The listing builds one solid part. Answer for the finished solid, in the listing's coordinates (mm). A direction names the side the tool comes from. Round coordinates to 2 decimals unless told otherwise and drop trailing zeros. Loops run counter-clockwise (first coordinate to the right, second up) from the corner with the lowest first, then second, coordinate; pieces in that order, holes last. Notation, with made-up numbers: M 70.5,58 L 90.5,58 A8 ccw 90.5,68 Z; hole C 86,67 d11. An arc over 180 degrees is marked long. Answer as a JSON object with one key per item and string values.
```python
from build123d import *

# Parameters (mm, degrees)
BOSS_EXTRUDE1_DEPTH     = 13
SKETCH6_W               = 6
SKETCH6_H               = 5
BOSS_EXTRUDE4_DEPTH     = 5.6
SKETCH16_W              = 6
SKETCH16_H              = 8
BOSS_EXTRUDE5_DEPTH     = 0.1
CUT_EXTRUDE6_DEPTH      = 4
CUT_EXTRUDE6_DEPTH_BACK = 3.6
SKETCH15_R              = 1.2
CUT_EXTRUDE7_DEPTH      = 8.7202
CUT_EXTRUDE8_START      = -0.2202
SKETCH19_W              = 6
SKETCH19_H              = 8
SKETCH19_R              = 1.2
CUT_EXTRUDE8_DEPTH      = 0.2202
SKETCH12_R              = 1.2
CUT_EXTRUDE5_DEPTH      = 6
CHAMFER1_SIZE           = 0.2
SKETCH21_R              = 1.2
BOSS_EXTRUDE6_DEPTH     = 2.5
SKETCH24_W              = 6
SKETCH24_H              = 5.5
CUT_EXTRUDE10_DEPTH     = 8.5
SKETCH25_W              = 6
SKETCH25_H              = 7
BOSS_EXTRUDE8_DEPTH     = 12.9
SKETCH26_W              = 6
SKETCH26_H              = 7.39
BOSS_EXTRUDE9_DEPTH     = 5
SKETCH27_W              = 6
SKETCH27_H              = 7.39
BOSS_EXTRUDE10_DEPTH    = 8
SKETCH28_R              = 1.2
CUT_EXTRUDE11_DEPTH     = 7.5
SKETCH30_R              = 1.2
CUT_EXTRUDE13_DEPTH     = 8
SKETCH31_W              = 7
SKETCH31_H              = 12.9
BOSS_EXTRUDE11_DEPTH    = 0.5
SKETCH32_W              = 7
SKETCH32_H              = 12.9
BOSS_EXTRUDE12_DEPTH    = 0.5
SKETCH33_W              = 0.5
SKETCH33_H              = 7.39
BOSS_EXTRUDE13_DEPTH    = 13
SKETCH34_R              = 1.2
CUT_EXTRUDE14_DEPTH     = 5


with BuildPart() as part:
    # Sketch1 → Boss-Extrude1 (new body)
    with BuildSketch(Plane.XY):
        Polygon((3, 3.05), (3, -2.253801214), (2.388188946, -2.95), (-2.388188946, -2.95), (-3, -2.253801214), (-3, 3.05), align=None)
    extrude(amount=BOSS_EXTRUDE1_DEPTH)

    # Sketch6 → Boss-Extrude4 (add)
    with BuildSketch(Plane(origin=(0, 3.05, 0), x_dir=(1, 0, 0), z_dir=(0, 1, 0))):
        with Locations((0, -2.5)):
            Rectangle(SKETCH6_W, SKETCH6_H)
    extrude(amount=BOSS_EXTRUDE4_DEPTH)

    # Sketch16 → Boss-Extrude5 (add)
    with BuildSketch(Plane(origin=(0, 3.05, 0), x_dir=(1, 0, 0), z_dir=(0, 1, 0))):
        with Locations((0, -9)):
            Rectangle(SKETCH16_W, SKETCH16_H)
    extrude(amount=BOSS_EXTRUDE5_DEPTH)

    # Sketch18 → Cut-Extrude6 (cut, two sides: drawn at the far end of the back side and taken through both)
    with BuildSketch(Plane(origin=(0, 0, 0), x_dir=(0, 0, -1), z_dir=(1, 0, 0)).offset(-CUT_EXTRUDE6_DEPTH_BACK)):
        with BuildLine():
            Line((-8.8572, -0.0702), (-12.8572, -0.0702))
            Line((-12.8572, -0.0702), (-13, -0.0702))
            Line((-13, -0.0702), (-13, -0.7))
            Line((-13, -0.7), (-12.8572, -0.7))
            Line((-12.8572, -0.7), (-12.7144, -0.7))
            add(Edge.make_bspline(
                [(-12.7144, -0.7), (-12.5198, -0.7), (-12.43, -0.9509)],
                knots=[0.103448276, 0.103448276, 0.103448276, 0.137931034, 0.137931034, 0.137931034], degree=2))
            add(Edge.make_bspline(
                [(-12.43, -0.9509), (-12.3594, -1.2388), (-12.13, -1.45), (-11.8572, -1.45)],
                knots=[0.137931034, 0.137931034, 0.137931034, 0.137931034, 0.172413793, 0.172413793, 0.172413793, 0.172413793], degree=3))
            add(Edge.make_bspline(
                [(-11.8572, -1.45), (-11.5844, -1.45), (-11.355, -1.2388), (-11.2844, -0.9509)],
                knots=[0.172413793, 0.172413793, 0.172413793, 0.172413793, 0.206896552, 0.206896552, 0.206896552, 0.206896552], degree=3))
            add(Edge.make_bspline(
                [(-11.2844, -0.9509), (-11.1946, -0.7), (-11, -0.7)],
                knots=[0.206896552, 0.206896552, 0.206896552, 0.24137931, 0.24137931, 0.24137931], degree=2))
            Line((-11, -0.7), (-10.8572, -0.7))
            Line((-10.8572, -0.7), (-10.7144, -0.7))
            add(Edge.make_bspline(
                [(-10.7144, -0.7), (-10.5198, -0.7), (-10.43, -0.9509)],
                knots=[0.310344828, 0.310344828, 0.310344828, 0.344827586, 0.344827586, 0.344827586], degree=2))
            add(Edge.make_bspline(
                [(-10.43, -0.9509), (-10.3594, -1.2388), (-10.13, -1.45), (-9.8572, -1.45)],
                knots=[0.344827586, 0.344827586, 0.344827586, 0.344827586, 0.379310345, 0.379310345, 0.379310345, 0.379310345], degree=3))
            add(Edge.make_bspline(
                [(-9.8572, -1.45), (-9.5844, -1.45), (-9.355, -1.2388), (-9.2844, -0.9509)],
                knots=[0.379310345, 0.379310345, 0.379310345, 0.379310345, 0.413793103, 0.413793103, 0.413793103, 0.413793103], degree=3))
            add(Edge.make_bspline(
                [(-9.2844, -0.9509), (-9.1946, -0.7), (-9, -0.7)],
                knots=[0.413793103, 0.413793103, 0.413793103, 0.448275862, 0.448275862, 0.448275862], degree=2))
            Line((-9, -0.7), (-8.8572, -0.7))
            Line((-8.8572, -0.7), (-8.7144, -0.7))
            add(Edge.make_bspline(
                [(-8.7144, -0.7), (-8.5198, -0.7), (-8.43, -0.9509)],
                knots=[0.517241379, 0.517241379, 0.517241379, 0.551724138, 0.551724138, 0.551724138], degree=2))
            add(Edge.make_bspline(
                [(-8.43, -0.9509), (-8.3594, -1.2388), (-8.13, -1.45), (-7.8572, -1.45)],
                knots=[0.551724138, 0.551724138, 0.551724138, 0.551724138, 0.586206897, 0.586206897, 0.586206897, 0.586206897], degree=3))
            add(Edge.make_bspline(
                [(-7.8572, -1.45), (-7.5844, -1.45), (-7.355, -1.2388), (-7.2844, -0.9509)],
                knots=[0.586206897, 0.586206897, 0.586206897, 0.586206897, 0.620689655, 0.620689655, 0.620689655, 0.620689655], degree=3))
            add(Edge.make_bspline(
                [(-7.2844, -0.9509), (-7.1946, -0.7), (-7, -0.7)],
                knots=[0.620689655, 0.620689655, 0.620689655, 0.655172414, 0.655172414, 0.655172414], degree=2))
            Line((-7, -0.7), (-6.8572, -0.7))
            Line((-6.8572, -0.7), (-6.7144, -0.7))
            add(Edge.make_bspline(
                [(-6.7144, -0.7), (-6.5198, -0.7), (-6.43, -0.9509)],
                knots=[0.724137931, 0.724137931, 0.724137931, 0.75862069, 0.75862069, 0.75862069], degree=2))
            add(Edge.make_bspline(
                [(-6.43, -0.9509), (-6.3594, -1.2388), (-6.13, -1.45), (-5.8572, -1.45)],
                knots=[0.75862069, 0.75862069, 0.75862069, 0.75862069, 0.793103448, 0.793103448, 0.793103448, 0.793103448], degree=3))
            add(Edge.make_bspline(
                [(-5.8572, -1.45), (-5.5844, -1.45), (-5.355, -1.2388), (-5.2844, -0.9509)],
                knots=[0.793103448, 0.793103448, 0.793103448, 0.793103448, 0.827586207, 0.827586207, 0.827586207, 0.827586207], degree=3))
            add(Edge.make_bspline(
                [(-5.2844, -0.9509), (-5.1946, -0.7), (-5, -0.7)],
                knots=[0.827586207, 0.827586207, 0.827586207, 0.862068966, 0.862068966, 0.862068966], degree=2))
            Line((-5, -0.7), (-5, -0.0702))
            Line((-5, -0.0702), (-8.8572, -0.0702))
        make_face()
    extrude(amount=CUT_EXTRUDE6_DEPTH + CUT_EXTRUDE6_DEPTH_BACK, mode=Mode.SUBTRACT)

    # Sketch15 → Cut-Extrude7 (cut)
    with BuildSketch(Plane(origin=(0, 8.65, 0), x_dir=(1, 0, 0), z_dir=(0, 1, 0))):
        with Locations(Location((0, -10.8572, 0), (0, 0, 180))):
            Circle(SKETCH15_R)
        with Locations(Location((0, -6.8572, 0), (0, 0, 180))):
            Circle(SKETCH15_R)
    extrude(amount=-CUT_EXTRUDE7_DEPTH, mode=Mode.SUBTRACT)

    # Sketch19 → Cut-Extrude8 (cut)
    with BuildSketch(Plane.XZ.offset(0.0702).offset(CUT_EXTRUDE8_START)):
        with Locations((0, 9)):
            Rectangle(SKETCH19_W, SKETCH19_H)
        with Locations(Location((0, 10.8572, 0), (0, 0, 180))):
            Circle(SKETCH19_R, mode=Mode.SUBTRACT)
        with Locations(Location((0, 6.8572, 0), (0, 0, 180))):
            Circle(SKETCH19_R, mode=Mode.SUBTRACT)
    extrude(amount=CUT_EXTRUDE8_DEPTH, mode=Mode.SUBTRACT)

    # Sketch12 → Cut-Extrude5 (cut)
    with BuildSketch(Plane.XY.offset(5)):
        with Locations((0, 5.85)):
            Circle(SKETCH12_R)
    extrude(amount=-CUT_EXTRUDE5_DEPTH, mode=Mode.SUBTRACT)

    # Chamfer1
    chamfer1_edges = [part.edges().sort_by_distance(p)[0] for p in [
        (-2.694094473, -2.601900607, 13),
        (0, -2.95, 13),
        (2.694094473, -2.601900607, 13),
        (3, 1.65, 13),
        (3, -1.476900607, 13),
        (-3, -1.476900607, 13),
        (-3, 1.65, 13),
    ]]
    chamfer(chamfer1_edges, length=CHAMFER1_SIZE)

    # Sketch21 → Boss-Extrude6 (add)
    with BuildSketch(Plane(origin=(0, 0, 0), x_dir=(-1, 0, 0), z_dir=(0, 0, -1))):
        Polygon((-2.388188946, -2.95), (2.388188946, -2.95), (3, -2.253801214), (3, 8.65), (-3, 8.65), (-3, -2.253801214), align=None)
        with Locations(Location((0, 5.85, 0), (0, 0, 180))):
            Circle(SKETCH21_R, mode=Mode.SUBTRACT)
    extrude(amount=BOSS_EXTRUDE6_DEPTH)

    # Sketch24 → Cut-Extrude10 (cut)
    with BuildSketch(Plane.XY.offset(5)):
        with Locations((0, 5.9)):
            Rectangle(SKETCH24_W, SKETCH24_H)
    extrude(amount=-CUT_EXTRUDE10_DEPTH, mode=Mode.SUBTRACT)

    # Sketch25 → Boss-Extrude8 (add)
    with BuildSketch(Plane(origin=(0, 3.15, 0), x_dir=(1, 0, 0), z_dir=(0, 1, 0))):
        with Locations((0, -1)):
            Rectangle(SKETCH25_W, SKETCH25_H)
    extrude(amount=BOSS_EXTRUDE8_DEPTH)

    # Sketch26 → Boss-Extrude9 (add)
    with BuildSketch(Plane(origin=(0, 0, -2.5), x_dir=(-1, 0, 0), z_dir=(0, 0, -1))):
        with Locations((0, 12.355)):
            Rectangle(SKETCH26_W, SKETCH26_H)
    extrude(amount=BOSS_EXTRUDE9_DEPTH)

    # Sketch27 → Boss-Extrude10 (add)
    with BuildSketch(Plane(origin=(0, 0, -7.5), x_dir=(-1, 0, 0), z_dir=(0, 0, -1))):
        with Locations((0, 12.355)):
            Rectangle(SKETCH27_W, SKETCH27_H)
    extrude(amount=BOSS_EXTRUDE10_DEPTH)

    # Sketch28 → Cut-Extrude11 (cut)
    with BuildSketch(Plane(origin=(0, 16.05, 0), x_dir=(1, 0, 0), z_dir=(0, 1, 0))):
        with Locations(Location((0, 11, 0), (0, 0, 180))):
            Circle(SKETCH28_R)
    extrude(amount=-CUT_EXTRUDE11_DEPTH, mode=Mode.SUBTRACT)

    # Sketch30 → Cut-Extrude13 (cut)
    with BuildSketch(Plane(origin=(0, 0, -2.5), x_dir=(-1, 0, 0), z_dir=(0, 0, -1))):
        with Locations((0, 5.9)):
            Circle(SKETCH30_R)
    extrude(amount=-CUT_EXTRUDE13_DEPTH, mode=Mode.SUBTRACT)

    # Sketch31 → Boss-Extrude11 (add)
    with BuildSketch(Plane(origin=(3, 0, 0), x_dir=(0, 0, -1), z_dir=(1, 0, 0))):
        with Locations((-1, 9.6)):
            Rectangle(SKETCH31_W, SKETCH31_H)
    extrude(amount=BOSS_EXTRUDE11_DEPTH)

    # Sketch32 → Boss-Extrude12 (add)
    with BuildSketch(Plane.ZY.offset(3)):
        with Locations((1, 9.6)):
            Rectangle(SKETCH32_W, SKETCH32_H)
    extrude(amount=BOSS_EXTRUDE12_DEPTH)

    # Sketch33 → Boss-Extrude13 (add)
    with BuildSketch(Plane(origin=(0, 0, -2.5), x_dir=(-1, 0, 0), z_dir=(0, 0, -1))):
        with Locations((-3.25, 12.355)):
            Rectangle(SKETCH33_W, SKETCH33_H)
        with Locations((3.25, 12.355)):
            Rectangle(SKETCH33_W, SKETCH33_H)
    extrude(amount=BOSS_EXTRUDE13_DEPTH)

    # Sketch34 → Cut-Extrude14 (cut)
    with BuildSketch(Plane(origin=(0, 16.05, 0), x_dir=(1, 0, 0), z_dir=(0, 1, 0))):
        with Locations(Location((0, 1, 0), (0, 0, 180))):
            Circle(SKETCH34_R)
    extrude(amount=-CUT_EXTRUDE14_DEPTH, mode=Mode.SUBTRACT)


solid = part.part
```
Item 1: Determine the mould class of faces 1 (the face through (0, 3.15, 9)), 2 (the face through (0.26, 12.41, -12.17)), 3 (the face through (0, 0, 5)) for opening direction Z: released by +Z, released by -Z, zero draft, split by the parting line, or undercut.
Values follow:
{"face 1": "zero draft", "face 2": "undercut", "face 3": "released by +Z"}
Item 2: The part is cut by section B-B (y = 6.25). Give the vertices of the cut face in (x, z).
Values follow:
{"outline": "M -3.5,-2.5 L -1.15,-2.5 L -1.15,4.5 L -3.5,4.5 Z; M 1.15,-2.5 L 3.5,-2.5 L 3.5,4.5 L 1.15,4.5 Z"}
Item 3: Flat-ended cylindrical pins translate along their axes: P1, Ø1.4, axis at x = 0, z = 6.86, coming from the +Y side; P2, Ø1.6, axis at y = 1.5, z = 4, coming from the -X side; P3, Ø6, axis at y = 2, z = 1.5, coming from the +X side; P4, Ø2, axis at x = 0.5, y = 9.5, coming from the +Z side. Find the tip coordinate at first contact, or state that the pin passes through.
Values follow:
{"P1": "y = -0.7", "P2": "x = -3", "P3": "x = 3.5", "P4": "z = 4.5"}
Item 4: Which of the six approach directions +Z, -Z, +X, -X, +Y, -Y give full straight-line access (tool end or side, diameter ignored) to faces 4 (the face through (0.26, 1.671, 5.686)), 5 (the face through (0, 8.66, -9)), 6 (the face through (3, 0.4, 5.3))?
Values follow:
{"face 4": "+Y", "face 5": "-Z, +X, -X, -Y", "face 6": "+Z, -Z, +X, -Y"}
Item 5: The part is cut by section C-C (y = 2.25). Give the vertices of the cut face in (x, z), then the cut area to 3 significant figures.
Values follow:
{"outline": "M -3,-2.5 L 3,-2.5 L 3,12.8 L 2.8,13 L -2.8,13 L -3,12.8 Z; hole C 0,6.86 d2.4; hole C 0,10.86 d2.4", "area": "83.9 mm^2"}
Item 6: The part is cut by section D-D (z = -11.75). Give the vertices of the cut face in (x, y), then the cut area to 3 significant figures.
Values follow:
{"outline": "M -3.5,8.66 L -0.94,8.66 L -0.94,16.05 L -3.5,16.05 Z; M 0.94,8.66 L 3.5,8.66 L 3.5,16.05 L 0.94,16.05 Z", "area": "37.9 mm^2"}
Item 7: The part is cut by section A-A (z = -1). Give the vertices of the cut face in (x, y).
Values follow:
{"outline": "M -3.5,3.15 L -3,3.15 L -3,-2.25 L -2.39,-2.95 L 2.39,-2.95 L 3,-2.25 L 3,3.15 L 3.5,3.15 L 3.5,16.05 L 1.2,16.05 L 1.2,11.05 L -1.2,11.05 L -1.2,16.05 L -3.5,16.05 Z; hole C 0,5.9 d2.4"}
Item 8: Straight lines are drawn through the part: line 1 (Z direction, x = 0, y = 3); line 2 (Z direction, x = 0, y = 12.15); line 3 (Z direction, x = -2.75, y = 13.5). For each, find the intervals that lie inside material, in ascending order.
Values follow:
{"line 1": "-2.5 to 5.66, 8.06 to 9.66, 12.06 to 13", "line 2": "-15.5 to -12.2, -9.8 to -2.2, 0.2 to 4.5", "line 3": "-15.5 to 4.5"}
